Verification items for the finished model (mm, model axes). Face numbers are marked on the shaded views. A direction names the side the tool comes from. Give positions to 0.01 mm unless a question says otherwise; leave off trailing zeros. Order: outer loops, then holes, each group sorted by start corner. A loop starts at its lowest first (then second) coordinate and runs counter-clockwise, first axis right, second up.
from build123d import *

# Parameters (mm, degrees)
SKETCH1_W           = 101.6
SKETCH1_H           = 101.6
BOSS_EXTRUDE1_DEPTH = 19.05
SKETCH2_R           = 18
SKETCH2_R_2         = 1.5
SKETCH2_R_3         = 13.25
SKETCH2_R_4         = 17.005
SKETCH2_R_5         = 12.7
BOSS_EXTRUDE2_DEPTH = 6.35
SKETCH3_W           = 101.6
SKETCH3_H           = 50.8
BOSS_EXTRUDE3_DEPTH = 6.35


with BuildPart() as part:
    # Sketch1 → Boss-Extrude1 (new body)
    with BuildSketch(Plane(origin=(0, 0, 0), x_dir=(1, 0, 0), z_dir=(0, 1, 0))):
        Rectangle(SKETCH1_W, SKETCH1_H)
    extrude(amount=BOSS_EXTRUDE1_DEPTH)

    # Sketch2 → Boss-Extrude2 (add)
    with BuildSketch(Plane(origin=(0, 19.05, 0), x_dir=(1, 0, 0), z_dir=(0, 1, 0))):
        with Locations((-25.4, 25.4)):
            Circle(SKETCH2_R)
        with Locations((-38.823393759, 33.15)):
            Circle(SKETCH2_R_2, mode=Mode.SUBTRACT)
        with Locations((-38.823393759, 17.65)):
            Circle(SKETCH2_R_2, mode=Mode.SUBTRACT)
        with Locations((-25.4, 9.9)):
            Circle(SKETCH2_R_2, mode=Mode.SUBTRACT)
        with Locations((-11.976606241, 17.65)):
            Circle(SKETCH2_R_2, mode=Mode.SUBTRACT)
        with Locations((-11.976606241, 33.15)):
            Circle(SKETCH2_R_2, mode=Mode.SUBTRACT)
        with Locations((-25.4, 40.9)):
            Circle(SKETCH2_R_2, mode=Mode.SUBTRACT)
        with Locations((-25.4, 25.4)):
            Circle(SKETCH2_R_3, mode=Mode.SUBTRACT)
        with Locations((25.4, 25.4)):
            Circle(SKETCH2_R_4)
        with Locations((11.976606241, 33.15)):
            Circle(SKETCH2_R_2, mode=Mode.SUBTRACT)
        with Locations((11.976606241, 17.65)):
            Circle(SKETCH2_R_2, mode=Mode.SUBTRACT)
        with Locations((25.4, 9.9)):
            Circle(SKETCH2_R_2, mode=Mode.SUBTRACT)
        with Locations((38.823393759, 17.65)):
            Circle(SKETCH2_R_2, mode=Mode.SUBTRACT)
        with Locations((38.823393759, 33.15)):
            Circle(SKETCH2_R_2, mode=Mode.SUBTRACT)
        with Locations((25.4, 40.9)):
            Circle(SKETCH2_R_2, mode=Mode.SUBTRACT)
        with Locations((25.4, 25.4)):
            Circle(SKETCH2_R_5, mode=Mode.SUBTRACT)
    extrude(amount=BOSS_EXTRUDE2_DEPTH)

    # Sketch3 → Boss-Extrude3 (add)
    with BuildSketch(Plane(origin=(0, 19.05, 0), x_dir=(1, 0, 0), z_dir=(0, 1, 0))):
        with Locations((0, -25.4)):
            Rectangle(SKETCH3_W, SKETCH3_H)
    extrude(amount=BOSS_EXTRUDE3_DEPTH)


solid = part.part
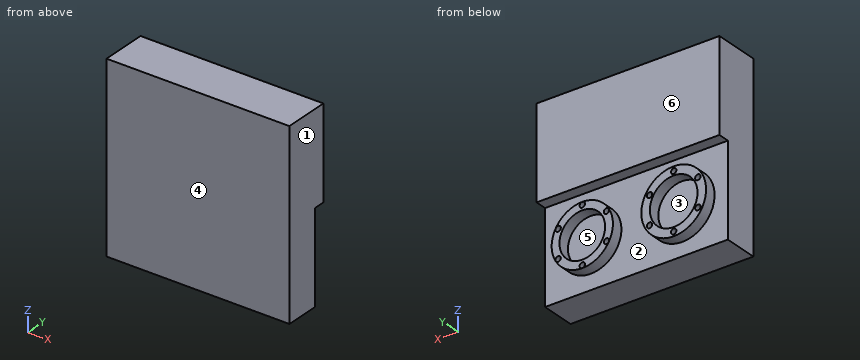
(1) Scan lines: line 1 (Z direction, x = -25.4, y = 22.75); line 2 (Z direction, x = 33.5, y = 21.5); line 3 (Z direction, x = 27.5, y = 23.5). Record each from-to range of solid material in increasing order.
Solved:
line 1: z = -43.4 to -42.4, -39.4 to -38.65, -12.15 to -11.4, -8.4 to -7.4, 0 to 50.8
line 2: z = -40.35 to -35.18, -15.62 to -10.45, 0 to 50.8
line 3: z = -42.27 to -37.93, -12.87 to -8.53, 0 to 50.8
(2) Set-up check for the marked faces 5 and 6: record each of +Z, -Z, +X, -X, +Y, -Y from which the full face is reachable in a straight line by a thin tool's end or side.
Solved:
face 5: +Y
face 6: +Z, -Z, +X, -X, +Y
(3) Release check for a two-part mould opening along X. For the marked faces 1, 2, 3 and 4 record: pulls with the +X half, pulls with the -X half, needs draft (parallel to the pull), parting line crosses it, or undercut.
Solved:
face 1: pulls with the +X half
face 2: undercut
face 3: undercut
face 4: needs draft
(4) Section check C-C, the plane x = -25.4. Enter the section's corners in (y, z).
Solved:
outline: (0, -50.8) - (19.05, -50.8) - (19.05, -43.4) - (25.4, -43.4) - (25.4, -42.4) - (19.05, -42.4) - (19.05, -39.4) - (25.4, -39.4) - (25.4, -38.65) - (19.05, -38.65) - (19.05, -12.15) - (25.4, -12.15) - (25.4, -11.4) - (19.05, -11.4) - (19.05, -8.4) - (25.4, -8.4) - (25.4, -7.4) - (19.05, -7.4) - (19.05, 0) - (25.4, 0) - (25.4, 50.8) - (0, 50.8) - close
(5) Section check B-B, the plane z = -25.4. Enter the section's corners in (x, y) (3 decimals), then the cut area to 3 significant figures.
Solved:
outline: (-50.8, 0) - (50.8, 0) - (50.8, 19.05) - (42.405, 19.05) - (42.405, 25.4) - (38.1, 25.4) - (38.1, 19.05) - (12.7, 19.05) - (12.7, 25.4) - (8.395, 25.4) - (8.395, 19.05) - (-7.4, 19.05) - (-7.4, 25.4) - (-12.15, 25.4) - (-12.15, 19.05) - (-38.65, 19.05) - (-38.65, 25.4) - (-43.4, 25.4) - (-43.4, 19.05) - (-50.8, 19.05) - close
area: 2,050 mm2
(6) Section check D-D, the plane z = -40.9. Enter the section's corners in (x, y).
Solved:
outline: (-50.8, 0) - (50.8, 0) - (50.8, 19.05) - (32.39, 19.05) - (32.39, 25.4) - (26.9, 25.4) - (26.9, 19.05) - (23.9, 19.05) - (23.9, 25.4) - (18.41, 25.4) - (18.41, 19.05) - (-16.25, 19.05) - (-16.25, 25.4) - (-23.9, 25.4) - (-23.9, 19.05) - (-26.9, 19.05) - (-26.9, 25.4) - (-34.55, 25.4) - (-34.55, 19.05) - (-50.8, 19.05) - close
(7) Section check A-A, the plane y = 23. Give the number of separate pieces and of enclosed holes in the cut face, then the cut area to 3 significant figures.
Solved:
separate pieces: 3
enclosed holes: 14
area: 5,940 mm2
(8) Go/stop test with flat-tipped pins: pin 1 (0.9 mm diameter, centred on x = -38.5, z = -17.5, fed in from +Y); pin 2 (3 mm diameter, centred on x = -17, y = 22.5, fed in from -Z) (3 decimals). Record where each tip stops, or that it passes through.
Solved:
pin 1: stops at y = 19.05
pin 2: stops at z = -42.025
